The listing builds one solid part. Answer for the finished solid, in the listing's coordinates (mm). A direction names the side the tool comes from. Give positions to 0.01 mm unless a question says otherwise; leave off trailing zeros. Write each loop counter-clockwise with the first axis right and the second up, starting at its lowest first coordinate (ties: lowest second). Pieces come first, ordered by that corner, then holes. Notation, with made-up numbers: (39.5, 77) -> (46.5, 77) arc R35 cw to (46.5, 113) -> close; hole circle Ø5 at (68, 87). An arc over 180 degrees is marked (long way). One line per question, with ' | ' between items.
from build123d import *

# Parameters (mm, degrees)
SKETCH2_R           = 1.5
BOSS_EXTRUDE1_DEPTH = 3
SKETCH4_W           = 1.5
SKETCH4_H           = 40
BOSS_EXTRUDE2_DEPTH = 48
CUT_EXTRUDE1_DEPTH  = 133.245982926
SKETCH6_R           = 18.5
BOSS_EXTRUDE3_DEPTH = 23
SKETCH7_R           = 16.25
BOSS_EXTRUDE4_DEPTH = 30
SKETCH8_R           = 6
BOSS_EXTRUDE5_DEPTH = 10
SKETCH9_R           = 34.15
BOSS_EXTRUDE6_DEPTH = 26


with BuildPart() as part:
    # Sketch2 → Boss-Extrude1 (new body)
    with BuildSketch(Plane(origin=(0, 0, 0), x_dir=(1, 0, 0), z_dir=(0, 1, 0))):
        with BuildLine():
            Line((57.5, -32), (-57.5, -32))
            ThreePointArc((-57.5, -32), (-58.914213562, -31.414213562), (-59.5, -30))
            Line((-59.5, -30), (-59.5, 30))
            ThreePointArc((-59.5, 30), (-58.914213562, 31.414213562), (-57.5, 32))
            Line((-57.5, 32), (57.5, 32))
            ThreePointArc((57.5, 32), (58.914213562, 31.414213562), (59.5, 30))
            Line((59.5, 30), (59.5, -30))
            ThreePointArc((59.5, -30), (58.914213562, -31.414213562), (57.5, -32))
        make_face()
        with Locations(Location((-56.5, 29, 0), (0, 0, 270))):
            Circle(SKETCH2_R, mode=Mode.SUBTRACT)
        with Locations(Location((-45.5, 26.25, 0), (0, 0, 270))):
            Circle(SKETCH2_R, mode=Mode.SUBTRACT)
        with Locations(Location((-25.5, 29, 0), (0, 0, 270))):
            Circle(SKETCH2_R, mode=Mode.SUBTRACT)
        with Locations(Location((-25.5, -29, 0), (0, 0, 90))):
            Circle(SKETCH2_R, mode=Mode.SUBTRACT)
        with Locations(Location((-45.5, -26.25, 0), (0, 0, 90))):
            Circle(SKETCH2_R, mode=Mode.SUBTRACT)
        with Locations(Location((-56.5, -29, 0), (0, 0, 90))):
            Circle(SKETCH2_R, mode=Mode.SUBTRACT)
        with Locations(Location((25.5, -29, 0), (0, 0, 270))):
            Circle(SKETCH2_R, mode=Mode.SUBTRACT)
        with Locations(Location((45.5, -26.25, 0), (0, 0, 270))):
            Circle(SKETCH2_R, mode=Mode.SUBTRACT)
        with Locations(Location((56.5, -29, 0), (0, 0, 270))):
            Circle(SKETCH2_R, mode=Mode.SUBTRACT)
        with Locations(Location((56.5, 29, 0), (0, 0, 90))):
            Circle(SKETCH2_R, mode=Mode.SUBTRACT)
        with Locations(Location((45.5, 26.25, 0), (0, 0, 90))):
            Circle(SKETCH2_R, mode=Mode.SUBTRACT)
        with Locations(Location((25.5, 29, 0), (0, 0, 90))):
            Circle(SKETCH2_R, mode=Mode.SUBTRACT)
        with BuildLine():
            Line((10, 28), (-10, 28))
            ThreePointArc((-10, 28), (-11.5, 26.5), (-10, 25))
            Line((-10, 25), (10, 25))
            ThreePointArc((10, 25), (11.5, 26.5), (10, 28))
        make_face(mode=Mode.SUBTRACT)
        with BuildLine():
            Line((-10, -25), (10, -25))
            ThreePointArc((10, -25), (11.5, -26.5), (10, -28))
            Line((10, -28), (-10, -28))
            ThreePointArc((-10, -28), (-11.5, -26.5), (-10, -25))
        make_face(mode=Mode.SUBTRACT)
    extrude(amount=BOSS_EXTRUDE1_DEPTH)

    # Sketch4 → Boss-Extrude2 (add)
    with BuildSketch(Plane.XZ):
        with Locations((-58.75, 0)):
            Rectangle(SKETCH4_W, SKETCH4_H)
    boss_extrude2 = extrude(amount=BOSS_EXTRUDE2_DEPTH)

    # Mirror3: Boss-Extrude2 across plane
    add(boss_extrude2.mirror(Plane(origin=(0, 0, 0), x_dir=(0, 0, 1), z_dir=(1, 0, 0))))

    # Sketch5 → Cut-Extrude1 (cut, through all)
    with BuildSketch(Plane.ZY.offset(59.5)):
        with BuildLine():
            ThreePointArc((-1.66e-07, -48), (-14.142135683, -42.142135565), (-20, -28))
            Line((-20, -28), (-20, -48))
            Line((-20, -48), (-1.66e-07, -48))
        make_face()
        with BuildLine():
            ThreePointArc((20, -28), (14.142135565, -42.142135683), (-1.66e-07, -48))
            Line((-1.66e-07, -48), (20, -48))
            Line((20, -48), (20, -28))
        make_face()
    extrude(amount=-CUT_EXTRUDE1_DEPTH, mode=Mode.SUBTRACT)

    # Sketch6 → Boss-Extrude3 (add)
    with BuildSketch(Plane(origin=(-58, 0, 0), x_dir=(0, 0, -1), z_dir=(1, 0, 0))):
        with Locations(Location((0, -28, 0), (0, 0, 180))):
            Circle(SKETCH6_R)
    boss_extrude3 = extrude(amount=BOSS_EXTRUDE3_DEPTH)

    # Sketch7 → Boss-Extrude4 (add)
    with BuildSketch(Plane(origin=(-35, 0, 0), x_dir=(0, 0, -1), z_dir=(1, 0, 0))):
        with Locations((0, -28)):
            Circle(SKETCH7_R)
    boss_extrude4 = extrude(amount=BOSS_EXTRUDE4_DEPTH)

    # Sketch8 → Boss-Extrude5 (add)
    with BuildSketch(Plane.ZY.offset(59.5)):
        with Locations(Location((0, -18, 0), (0, 0, 180))):
            Circle(SKETCH8_R)
    boss_extrude5 = extrude(amount=BOSS_EXTRUDE5_DEPTH)

    # Sketch9 → Boss-Extrude6 (add)
    with BuildSketch(Plane.ZY.offset(69.5)):
        with Locations(Location((0, -18, 0), (0, 0, 180))):
            Circle(SKETCH9_R)
    boss_extrude6 = extrude(amount=BOSS_EXTRUDE6_DEPTH)

    # Mirror7: Boss-Extrude3, Boss-Extrude4, Boss-Extrude5, Boss-Extrude6 across plane
    add(boss_extrude3.mirror(Plane(origin=(0, 0, 0), x_dir=(0, 0, 1), z_dir=(1, 0, 0))))
    add(boss_extrude4.mirror(Plane(origin=(0, 0, 0), x_dir=(0, 0, 1), z_dir=(1, 0, 0))))
    add(boss_extrude5.mirror(Plane(origin=(0, 0, 0), x_dir=(0, 0, 1), z_dir=(1, 0, 0))))
    add(boss_extrude6.mirror(Plane(origin=(0, 0, 0), x_dir=(0, 0, 1), z_dir=(1, 0, 0))))


solid = part.part
Item 1: Flat-ended cylindrical pins translate along their axes: pin 1 (1.6 mm diameter, centred on x = -58.5, y = -14, fed in from -Z); pin 2 (10 mm diameter, centred on x = -48, z = 9, fed in from -Y); pin 3 (3.5 mm diameter, centred on x = 56.5, z = 29, fed in from +Y). Find the tip coordinate at first contact, or state that the pin passes through.
Answers below:
pin 1: z = -20 | pin 2: y = -46.06 | pin 3: y = 3
Item 2: Find section C-C (z = 14). Count the separate pieces of the cut face and the enclosed holes in it, then the cut area to 3 significant figures.
Answers below:
separate pieces: 3 | enclosed holes: 0 | area: 5,830 mm²
Item 3: Find section D-D (x = -77.5). Write down the section's boundary in (y, z).
Answers below:
outline: circle Ø68.3 at (-18, 0)
Item 4: Find section B-B (x = 31). Write down the section's boundary in (y, z), then the cut area to 3 significant figures.
Answers below:
outline: circle Ø32.5 at (-28, 0); (0, -32) -> (3, -32) -> (3, 32) -> (0, 32) -> close | area: 1,020 mm²
Item 5: Find section A-A (z = -22). Write down the section's boundary in (x, y), then the cut area to 3 significant figures.
Answers below:
outline: (-95.5, -44.12) -> (-69.5, -44.12) -> (-69.5, 8.12) -> (-95.5, 8.12) -> close; (-59.5, 0) -> (59.5, 0) -> (59.5, 3) -> (-59.5, 3) -> close; (69.5, -44.12) -> (95.5, -44.12) -> (95.5, 8.12) -> (69.5, 8.12) -> close | area: 3,070 mm²
Item 6: Consider line 1 (X direction, y = -5, z = -4); line 2 (X direction, y = 2, z = 29); line 3 (X direction, y = -29, z = -7.5). Determine where each line is inside the solid, lowest interval first. Write a range as [from, to].
Answers below:
line 1: [-95.5, -69.5], [-59.5, -58], [58, 59.5], [69.5, 95.5] | line 2: [-59.5, -58], [-55, -27], [-24, 24], [27, 55], [58, 59.5] | line 3: [-95.5, -69.5], [-59.5, -5], [5, 59.5], [69.5, 95.5]
Item 7: Determine the mould class of faces 6 (the face through (1, 0, 0)), 7 (the face through (-46.661, -46.343, -2.408)), 8 (the face through (-64.43, -19.802, -5.723)), 9 (the face through (-5, -28, 0)) for opening direction Y: pulls with the +Y half, pulls with the -Y half, needs draft (parallel to the pull), parting line crosses it, or undercut.
Answers below:
face 6: undercut | face 7: undercut | face 8: parting line crosses it | face 9: needs draft
Item 8: A tool of negligible diameter and unlimited length cuts with its end or side. For faces 1 (the face through (46.661, -46.343, -2.408)), 2 (the face through (-95.5, -18, 0)), 3 (the face through (95.5, -18, 0)), 4 (the face through (1, 3, 0)), 5 (the face through (5, -28, 0)), from which of +Z, -Z, +X, -X, +Y, -Y can it reach the whole face along a straight path? Write none if from no direction.
Answers below:
face 1: none | face 2: +Z, -Z, -X, +Y, -Y | face 3: +Z, -Z, +X, +Y, -Y | face 4: +Z, -Z, +Y | face 5: +Z, -Z, -Y
